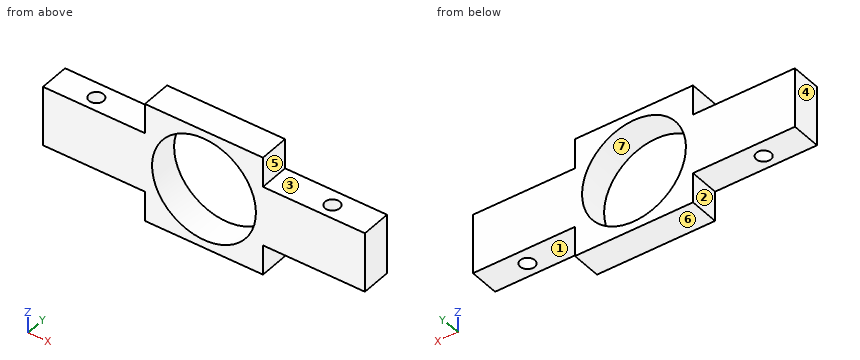
from build123d import *

# Parameters (mm, degrees)
SKETCH1_R               = 11
BOSS_EXTRUDE1_DEPTH     = 6.35
CUT_EXTRUDE1_DEPTH      = 40.56454347
CUT_EXTRUDE1_DEPTH_BACK = 40.56454347
SKETCH2_R               = 1.55


with BuildPart() as part:
    # Sketch1 → Boss-Extrude1 (new body)
    with BuildSketch(Plane(origin=(0, 0, 0), x_dir=(1, 0, 0), z_dir=(0, 1, 0))):
        Polygon((-34.09, 6.35), (-12.5, 6.35), (-12.5, 12.7), (12.5, 12.7), (12.5, 6.35), (34.09, 6.35), (34.09, -6.35), (12.5, -6.35), (12.5, -12.7), (-12.5, -12.7), (-12.5, -6.35), (-34.09, -6.35), align=None)
        with Locations(Location((0, 0, 0), (0, 0, 270))):
            Circle(SKETCH1_R, mode=Mode.SUBTRACT)
    extrude(amount=BOSS_EXTRUDE1_DEPTH)

    # Sketch2 → Cut-Extrude1 (cut, two sides: drawn at the far end of the back side and taken through both)
    with BuildSketch(Plane(origin=(0, 0, -6.35), x_dir=(-1, 0, 0), z_dir=(0, 0, -1)).offset(-CUT_EXTRUDE1_DEPTH_BACK)):
        with Locations((25, 3)):
            Circle(SKETCH2_R)
        with Locations((-25, 3)):
            Circle(SKETCH2_R)
    extrude(amount=CUT_EXTRUDE1_DEPTH + CUT_EXTRUDE1_DEPTH_BACK, mode=Mode.SUBTRACT)


solid = part.part
The listing builds one solid part. Answer for the finished solid, in the listing's coordinates (mm). Face numbers are marked on the shaded views. A direction names the side the tool comes from. Give positions to 0.01 mm unless a question says otherwise; leave off trailing zeros. Write each loop counter-clockwise with the first axis right and the second up, starting at its lowest first coordinate (ties: lowest second). Pieces come first, ordered by that corner, then holes. Notation, with made-up numbers: (85.5, 38.25) - (90.5, 38.25) arc R17 ccw to (90.5, 44.25) - close; hole circle Ø11 at (-2.75, 4.5). An arc over 180 degrees is marked (long way). One line per question, with ' | ' between items. Start each with the question number.
1. Determine the mould class of the marked faces 4, 5, 6 and 7 for opening direction X: +X half, -X half, draft (parallel to the pull), parting line (faces both ways), or undercut.
2. Given P1, Ø1.9, axis at y = 2, z = -9.5, coming from the +X side; P2, Ø1.9, axis at x = 26.5, y = 3, coming from the +Z side; P3, Ø3, axis at x = -27, y = 1, coming from the -Z side, each flat-ended and moving along its own axis, determine where each tip first touches the part or whether it passes through.
3. Section D-D, the plane z = 5.5 is taken. Determine the outline of the cut face in (x, y), then the cut area to 3 significant figures.
4. Section A-A, the plane y = 3 is taken. Determine the outline of the cut face in (x, z), then the cut area to 3 significant figures.
5. Section C-C, the plane x = -25 is taken. Determine the outline of the cut face in (y, z).
6. Straight lines are drawn through the part: line 1 (Y direction, x = -25, z = 2.25); line 2 (X direction, y = 5, z = -0.5); line 3 (X direction, y = 3.5, z = 2). For each, find the intervals that lie inside material, in ascending order.
7. For the marked faces 1, 2 and 3, determine the directions among +Z, -Z, +X, -X, +Y, -Y from which every point of the face is accessible in a straight line to the end or side of a thin tool.
8. Section B-B, the plane z = 0 is taken. Determine the outline of the cut face in (x, y).
Result:
1) face 4: -X half | face 5: +X half | face 6: draft | face 7: undercut
2) P1: stops at x = 12.5 | P2: stops at z = 6.35 | P3: stops at z = -6.35
3) outline: (-34.09, 0) - (-9.53, 0) - (-9.53, 6.35) - (-34.09, 6.35) - close; (9.53, 0) - (34.09, 0) - (34.09, 6.35) - (9.53, 6.35) - close; hole circle Ø3.1 at (-25, 3); hole circle Ø3.1 at (25, 3) | area: 297 mm2
4) outline: (-34.09, -6.35) - (-26.55, -6.35) - (-26.55, 6.35) - (-34.09, 6.35) - close; (-23.45, -6.35) - (-12.5, -6.35) - (-12.5, -12.7) - (12.5, -12.7) - (12.5, -6.35) - (23.45, -6.35) - (23.45, 6.35) - (12.5, 6.35) - (12.5, 12.7) - (-12.5, 12.7) - (-12.5, 6.35) - (-23.45, 6.35) - close; (26.55, -6.35) - (34.09, -6.35) - (34.09, 6.35) - (26.55, 6.35) - close; hole circle Ø22 at (0, 0) | area: 725 mm2
5) outline: (0, -6.35) - (1.45, -6.35) - (1.45, 6.35) - (0, 6.35) - close; (4.55, -6.35) - (6.35, -6.35) - (6.35, 6.35) - (4.55, 6.35) - close
6) line 1: y = 0 to 1.45, 4.55 to 6.35 | line 2: x = -34.09 to -10.99, 10.99 to 34.09 | line 3: x = -34.09 to -26.47, -23.53 to -10.82, 10.82 to 23.53, 26.47 to 34.09
7) face 1: -Z, +X, +Y, -Y | face 2: -Z, -X, +Y, -Y | face 3: +Z, +X, +Y, -Y
8) outline: (-34.09, 0) - (-11, 0) - (-11, 6.35) - (-34.09, 6.35) - close; (11, 0) - (34.09, 0) - (34.09, 6.35) - (11, 6.35) - close; hole circle Ø3.1 at (-25, 3); hole circle Ø3.1 at (25, 3)
